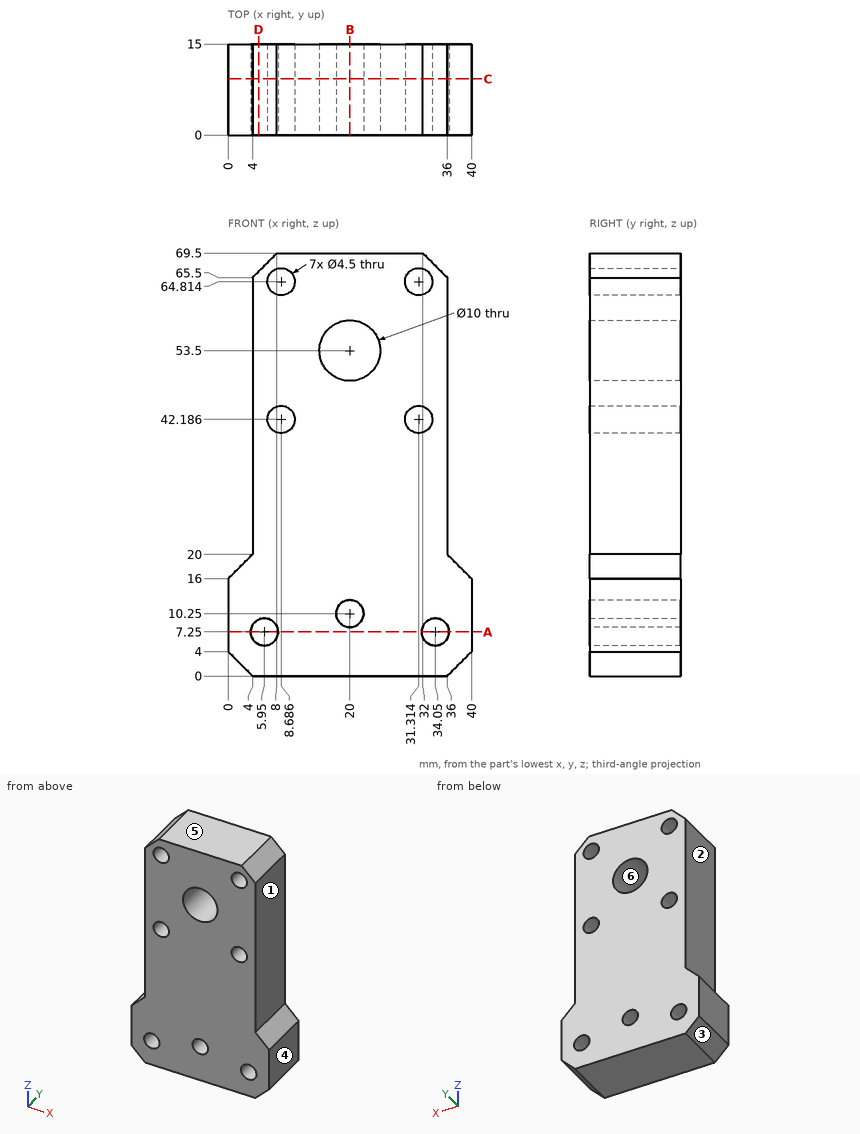
Answer from the drawing. Dimensions are ordinates in mm from the lowest x, y and z of the part. A direction names the side the tool comes from. Round coordinates to 2 decimals unless told otherwise and drop trailing zeros. Loops run counter-clockwise (first coordinate to the right, second up) from the corner with the lowest first, then second, coordinate; pieces in that order, holes last. Notation, with made-up numbers: (-3, -22) - (27, -22) arc R19 cw to (27, 12) - close; hole circle Ø1 at (-19.75, -0.5). An arc over 180 degrees is marked (long way). Return JSON: item names as keys, results as strings. Group by question number.
1. Which of the six approach directions +Z, -Z, +X, -X, +Y, -Y give full straight-line access (tool end or side, diameter ignored) to the marked faces 1, 2 and 3?
2. The mould has two halves that part along X. Classify the marked faces 4, 5 and 6: pulls with the +X half, pulls with the -X half, needs draft (parallel to the pull), parting line crosses it, or undercut.
3. The part is cut by section D-D on x = 5. Determine the outline of the cut face in (y, z).
4. The part is cut by section C-C on y = 9.25. State how many separate pieces and enclosed holes the cut face has, then the cut area to 3 significant figures.
5. Each of these flat-tipped pins is pushed along its axis until it touches: P1, Ø2.5, axis at x = 5.95, z = 7.25, coming from the -Y side; P2, Ø1.5, axis at y = 3.5, z = 44.5, coming from the +X side; P3, Ø4.5, axis at y = 8.5, z = 42, coming from the -X side. Where does it stop, or does it pass through?
6. Consider probe 1 along Z at (x, y) = (32, 12) (1 decimal); probe 2 along Z at (x, y) = (7, 3.25) (1 decimal); probe 3 along Z at (x, y) = (18, 13.75) (1 decimal). Determine where each line is inside the solid, lowest interval first.
7. The part is cut by section A-A on z = 7.25. Determine the outline of the cut face in (x, y), then the cut area to 3 significant figures.
8. The part is cut by section B-B on x = 20. Determine the outline of the cut face in (y, z), then the cut area to 3 significant figures.
Resolved:
{
 "1": {"face 1": "+Z, +X, +Y, -Y", "face 2": "+Z, -X, +Y, -Y", "face 3": "-Z, -X, +Y, -Y"},
 "2": {"face 4": "pulls with the +X half", "face 5": "needs draft", "face 6": "undercut"},
 "3": {"outline": "(0, 0) - (15, 0) - (15, 5.21) - (0, 5.21) - close; (0, 9.29) - (15, 9.29) - (15, 66.5) - (0, 66.5) - close"},
 "4": {"separate pieces": "1", "enclosed holes": "8", "area": "2,150 mm²"},
 "5": {"P1": "passes through", "P2": "stops at x = 36", "P3": "stops at x = 4"},
 "6": {"probe 1": "z = 0 to 6.3, 8.2 to 40, 44.3 to 62.7, 67 to 69.5", "probe 2": "z = 0 to 5.3, 9.2 to 40.7, 43.7 to 63.3, 66.3 to 68.5", "probe 3": "z = 0 to 9.2, 11.3 to 48.9, 58.1 to 69.5"},
 "7": {"outline": "(0, 0) - (3.7, 0) - (3.7, 15) - (0, 15) - close; (8.2, 0) - (31.8, 0) - (31.8, 15) - (8.2, 15) - close; (36.3, 0) - (40, 0) - (40, 15) - (36.3, 15) - close", "area": "465 mm²"},
 "8": {"outline": "(0, 0) - (15, 0) - (15, 8) - (0, 8) - close; (0, 12.5) - (15, 12.5) - (15, 48.5) - (0, 48.5) - close; (0, 58.5) - (15, 58.5) - (15, 69.5) - (0, 69.5) - close", "area": "825 mm²"}
}
